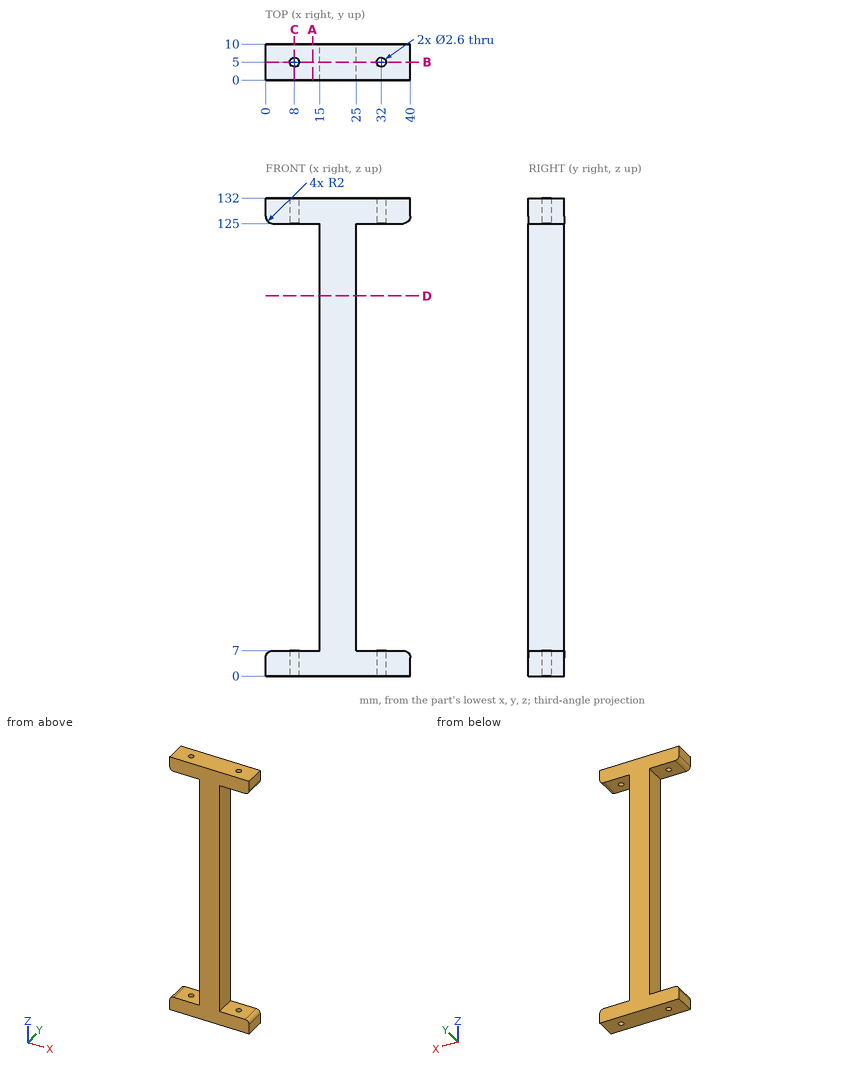
Source: three-view drawing plus pictorial views. Frame: mm from the lowest corner of the part. Give positions to 0.01 mm unless a question says otherwise; leave off trailing zeros. Write each loop counter-clockwise with the first axis right and the second up, starting at its lowest first coordinate (ties: lowest second). Pieces come first, ordered by that corner, then holes.
(1) Cut plane C-C, the plane x = 8. Return loops of the section in (y, z), then the cut area to 3 significant figures.
(2) Ray query, line 1 (X direction, y = 5, z = 126.75); line 2 (Z direction, x = 33, y = 9); line 3 (X direction, y = 5, z = 126.5). Return the intervals inside material, ascending.
(3) Cut plane D-D, the plane z = 105. Return loops of the section in (x, y), then the cut area to 3 significant figures.
(4) Cut plane A-A, the plane x = 13. Return loops of the section in (y, z).
(5) First-contact query: P1, Ø1.5, axis at y = 3, z = 81.5, coming from the +X side; P2, Ø1.6, axis at x = 32, y = 5, coming from the +Z side. Flat tips, straight axial feed; report the tip coordinate or a pass-through.
(6) Cut plane B-B, the plane y = 5. Give the number of separate pieces and of enclosed holes in the cut face, then the cut area to 3 significant figures.
Values follow:
1. outline: (0, 0) - (3.7, 0) - (3.7, 7) - (0, 7) - close; (0, 125) - (3.7, 125) - (3.7, 132) - (0, 132) - close; (6.3, 0) - (10, 0) - (10, 7) - (6.3, 7) - close; (6.3, 125) - (10, 125) - (10, 132) - (6.3, 132) - close
1. area: 104 mm2
2. line 1: x = 0.02 to 6.7, 9.3 to 30.7, 33.3 to 39.98
2. line 2: z = 0 to 7, 125 to 132
2. line 3: x = 0.06 to 6.7, 9.3 to 30.7, 33.3 to 39.94
3. outline: (15, 0) - (25, 0) - (25, 10) - (15, 10) - close
3. area: 100 mm2
4. outline: (0, 0) - (10, 0) - (10, 7) - (0, 7) - close; (0, 125) - (10, 125) - (10, 132) - (0, 132) - close
5. P1: stops at x = 25
5. P2: passes through
6. separate pieces: 5
6. enclosed holes: 0
6. area: 1,660 mm2
